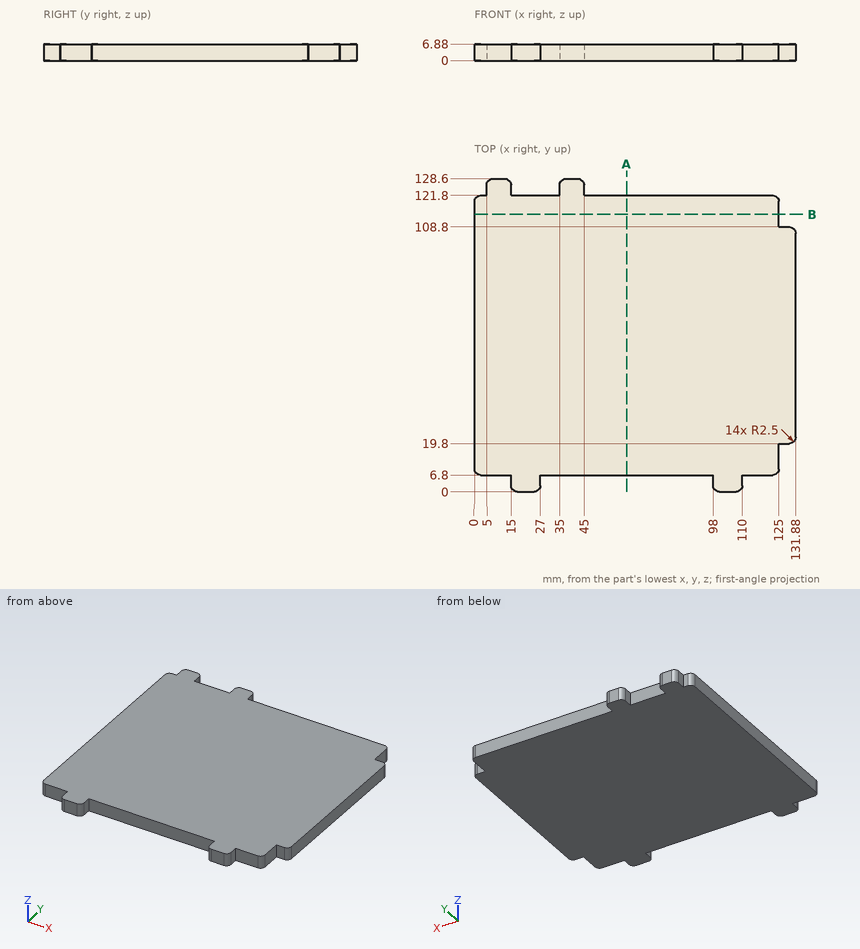
Print and shaded views of the part. All mm, measured from the part's lowest x, y and z. Round coordinates to 2 decimals unless told otherwise and drop trailing zeros. Write each loop counter-clockwise with the first axis right and the second up, starting at its lowest first coordinate (ties: lowest second). Pieces come first, ordered by that corner, then holes. Notation, with made-up numbers: M 40.5,18 L 97.5,18 A19 cw 97.5,33 Z; hole C 20.25,58.25 d5. An arc over 180 degrees is marked long. One line per question, with ' | ' between items.
(1) Saw through at A-A on x = 62.5. Write the cut outline in (y, z), then the cut area to 3 significant figures.
Answer key:
outline: M 6.8,0 L 121.8,0 L 121.8,6.88 L 6.8,6.88 Z | area: 791 mm^2
(2) Saw through at B-B on y = 114. Write the cut outline in (x, z).
Answer key:
outline: M 0,0 L 125,0 L 125,6.88 L 0,6.88 Z
(3) Probe line 1 along X through (y, z) = (18.5, 5.75); line 2 along Y through (x, z) = (101, 3.5); line 3 along Y through (x, z) = (72, 1.5). List the from-to ranges inside material, lowest first.
Answer key:
line 1: x = 0 to 125 | line 2: y = 0 to 121.8 | line 3: y = 6.8 to 121.8
(4) Pin check, flat tips, straight feed: pin 1 (2 mm diameter, centred on y = 15, z = 4.5, fed in from +X); pin 2 (3 mm diameter, centred on x = 62.5, z = 5, fed in from +Y); pin 3 (2 mm diameter, centred on y = 125, z = 5, fed in from -X). Stop position of each tip, or through.
Answer key:
pin 1: stops at x = 125 | pin 2: stops at y = 121.8 | pin 3: stops at x = 5
